from build123d import *

# Parameters (mm, degrees)
SKIZZE1_W                       = 1453
SKIZZE1_H                       = 700
SKIZZE1_W_2                     = 1333
SKIZZE1_H_2                     = 580
AUFSATZ_LINEAR_AUSTRAGEN1_DEPTH = 60
VERRUNDUNG1_R                   = 10
SKIZZE2_W                       = 300
SKIZZE2_H                       = 60
AUFSATZ_LINEAR_AUSTRAGEN2_DEPTH = 120
VERRUNDUNG3_R                   = 10
VERRUNDUNG4_R                   = 10
SKIZZE3_R                       = 8.75
SCHNITT_LINEAR_AUSTRAGEN1_DEPTH = 120
SKIZZE4_W                       = 80
SKIZZE4_H                       = 40
AUFSATZ_LINEAR_AUSTRAGEN3_DEPTH = 25


with BuildPart() as part:
    # Skizze1 → Aufsatz-Linear austragen1 (new, symmetric)
    with BuildSketch(Plane(origin=(0, 0, 0), x_dir=(1, 0, 0), z_dir=(0, 1, 0))):
        Rectangle(SKIZZE1_W, SKIZZE1_H)
        Rectangle(SKIZZE1_W_2, SKIZZE1_H_2, mode=Mode.SUBTRACT)
    extrude(amount=AUFSATZ_LINEAR_AUSTRAGEN1_DEPTH, both=True)

    # Verrundung1
    verrundung1_edges = [part.edges().sort_by_distance(p)[0] for p in [
        (726.5, 60, 0),
        (0, 60, -350),
        (-666.5, -60, 0),
        (0, -60, 290),
        (666.5, -60, 0),
        (0, -60, -290),
        (-666.5, 60, 0),
        (0, 60, 290),
        (666.5, 60, 0),
        (0, 60, -290),
        (-726.5, 60, 0),
        (0, -60, -350),
        (726.5, -60, 0),
        (0, -60, 350),
        (-726.5, -60, 0),
        (0, 60, 350),
    ]]
    fillet(verrundung1_edges, radius=VERRUNDUNG1_R)

    # Skizze2 → Aufsatz-Linear austragen2 (add)
    with BuildSketch(Plane.XZ.offset(60)):
        with Locations((-576.5, 320)):
            Rectangle(SKIZZE2_W, SKIZZE2_H)
        with Locations((576.5, 320)):
            Rectangle(SKIZZE2_W, SKIZZE2_H)
        with Locations((576.5, -320)):
            Rectangle(SKIZZE2_W, SKIZZE2_H)
        with Locations((-576.5, -320)):
            Rectangle(SKIZZE2_W, SKIZZE2_H)
    extrude(amount=AUFSATZ_LINEAR_AUSTRAGEN2_DEPTH)

    # Verrundung3
    verrundung3_edges = [part.edges().sort_by_distance(p)[0] for p in [
        (576.5, -180, 290),
        (576.5, -180, -290),
        (576.5, -180, -350),
        (-576.5, -180, -350),
        (-576.5, -180, -290),
        (-576.5, -180, 290),
        (-576.5, -180, 350),
        (576.5, -180, 350),
    ]]
    fillet(verrundung3_edges, radius=VERRUNDUNG3_R)

    # Verrundung4
    # the kernel refuses this fillet: 10 mm, written as the material it adds along each edge
    # the kernel refuses this fillet: 10 mm, written as the material it takes off along each edge
    with BuildSketch(Plane(origin=(691.5, -60, -290), x_dir=(0, 0, -1), z_dir=(1, 0, 0)), Plane(origin=(-691.5, -60, -290), x_dir=(0, -1, 0), z_dir=(-1, 0, 0))) as verrundung4_2_piece_1:
        with BuildLine():
            CenterArc((VERRUNDUNG4_R, -VERRUNDUNG4_R), VERRUNDUNG4_R, 90, 90)
            Line((0, -VERRUNDUNG4_R), (0, 0))
            Line((0, 0), (VERRUNDUNG4_R, 0))
        make_face()
    extrude(amount=60, mode=Mode.SUBTRACT)
    with BuildSketch(Plane(origin=(401.5, -60, -290), x_dir=(0, 0, -1), z_dir=(1, 0, 0)), Plane(origin=(-401.5, -60, -290), x_dir=(0, -1, 0), z_dir=(-1, 0, 0))) as verrundung4_2_piece_2:
        with BuildLine():
            CenterArc((VERRUNDUNG4_R, -VERRUNDUNG4_R), VERRUNDUNG4_R, 90, 90)
            Line((0, -VERRUNDUNG4_R), (0, 0))
            Line((0, 0), (VERRUNDUNG4_R, 0))
        make_face()
    extrude(amount=300, mode=Mode.SUBTRACT)
    with BuildSketch(Plane(origin=(751.5, -60, -350), x_dir=(0, 0, 1), z_dir=(-1, 0, 0)), Plane(origin=(-751.5, -60, 350), x_dir=(0, 0, -1), z_dir=(1, 0, 0))) as verrundung4_2_piece_3:
        with BuildLine():
            CenterArc((VERRUNDUNG4_R, -VERRUNDUNG4_R), VERRUNDUNG4_R, 90, 90)
            Line((0, -VERRUNDUNG4_R), (0, 0))
            Line((0, 0), (VERRUNDUNG4_R, 0))
        make_face()
    extrude(amount=350, mode=Mode.SUBTRACT)
    with BuildSketch(Plane(origin=(-751.5, -60, -350), x_dir=(0, 0, 1), z_dir=(1, 0, 0)), Plane(origin=(751.5, -60, 350), x_dir=(0, 0, -1), z_dir=(-1, 0, 0))) as verrundung4_2_piece_4:
        with BuildLine():
            CenterArc((VERRUNDUNG4_R, VERRUNDUNG4_R), VERRUNDUNG4_R, 180, 90)
            Line((0, VERRUNDUNG4_R), (0, 0))
            Line((0, 0), (VERRUNDUNG4_R, 0))
        make_face()
    extrude(amount=350, mode=Mode.SUBTRACT)
    with BuildSketch(Plane(origin=(-691.5, -60, 290), x_dir=(0, -1, 0), z_dir=(-1, 0, 0)), Plane(origin=(691.5, -60, 290), x_dir=(0, 0, 1), z_dir=(1, 0, 0))) as verrundung4_2_piece_5:
        with BuildLine():
            CenterArc((VERRUNDUNG4_R, VERRUNDUNG4_R), VERRUNDUNG4_R, 180, 90)
            Line((0, VERRUNDUNG4_R), (0, 0))
            Line((0, 0), (VERRUNDUNG4_R, 0))
        make_face()
    extrude(amount=60, mode=Mode.SUBTRACT)
    with BuildSketch(Plane(origin=(-401.5, -60, 290), x_dir=(0, -1, 0), z_dir=(-1, 0, 0)), Plane(origin=(401.5, -60, 290), x_dir=(0, 0, 1), z_dir=(1, 0, 0))) as verrundung4_2_piece_6:
        with BuildLine():
            CenterArc((VERRUNDUNG4_R, VERRUNDUNG4_R), VERRUNDUNG4_R, 180, 90)
            Line((0, VERRUNDUNG4_R), (0, 0))
            Line((0, 0), (VERRUNDUNG4_R, 0))
        make_face()
    extrude(amount=300, mode=Mode.SUBTRACT)

    # Skizze3 → Schnitt-Linear austragen1 (cut)
    with BuildSketch(Plane.XZ.offset(180)):
        with Locations(Location((-619.5, 320, 0), (0, 0, 270))):
            Circle(SKIZZE3_R)
        with Locations(Location((-619.5, -320, 0), (0, 0, 270))):
            Circle(SKIZZE3_R)
        with Locations(Location((619.5, 320, 0), (0, 0, 270))):
            Circle(SKIZZE3_R)
        with Locations(Location((619.5, -320, 0), (0, 0, 270))):
            Circle(SKIZZE3_R)
    extrude(amount=-SCHNITT_LINEAR_AUSTRAGEN1_DEPTH, mode=Mode.SUBTRACT)

    # Skizze4 → Aufsatz-Linear austragen3 (add)
    with BuildSketch(Plane.XZ.offset(180)):
        with Locations((-551.5, 320)):
            Rectangle(SKIZZE4_W, SKIZZE4_H)
        with Locations((551.5, 320)):
            Rectangle(SKIZZE4_W, SKIZZE4_H)
        with Locations((551.5, -320)):
            Rectangle(SKIZZE4_W, SKIZZE4_H)
        with Locations((-551.5, -320)):
            Rectangle(SKIZZE4_W, SKIZZE4_H)
    extrude(amount=AUFSATZ_LINEAR_AUSTRAGEN3_DEPTH)


solid = part.part
Verification items for the finished model (mm, model axes). A direction names the side the tool comes from. Coordinates: 2 decimals unless noted, no trailing zeros. Loops run counter-clockwise (first coordinate to the right, second up) from the corner with the lowest first, then second, coordinate; pieces in that order, holes last. Notation, with made-up numbers: (23, 7.25) -> (43, 7.25) arc R21 cw to (43, 13.25) -> close; hole circle Ø3 at (81, 36). An arc over 180 degrees is marked (long way). Answer as CSV lines item,"result".
1) Depth check by flat-ended pin: pin 1 (7.5 mm diameter, centred on y = -196, z = -321.5, fed in from -X); pin 2 (14 mm diameter, centred on x = -617.5, z = -317.5, fed in from -Y); pin 3 (20 mm diameter, centred on y = -194, z = 321, fed in from +X). Enter the tip coordinate at first touch or a pass-through.
Found:
pin 1,"stops at x = -591.5"
pin 2,"stops at y = -180"
pin 3,"stops at x = 591.5"
2) Cross-section at C-C, the plane z = -50.5. Record the cut outline in (x, y).
Found:
outline,"(-726.5, -50) arc R10 ccw to (-716.5, -60) -> (-676.5, -60) arc R10 ccw to (-666.5, -50) -> (-666.5, 50) arc R10 ccw to (-676.5, 60) -> (-716.5, 60) arc R10 ccw to (-726.5, 50) -> close; (666.5, -50) arc R10 ccw to (676.5, -60) -> (716.5, -60) arc R10 ccw to (726.5, -50) -> (726.5, 50) arc R10 ccw to (716.5, 60) -> (676.5, 60) arc R10 ccw to (666.5, 50) -> close"
3) Cross-section at A-A, the plane y = -151.5. Record the cut outline in (x, z), then the cut area to 3 significant figures.
Found:
outline,"(-726.5, -350) -> (-426.5, -350) -> (-426.5, -290) -> (-726.5, -290) -> close; (-726.5, 290) -> (-426.5, 290) -> (-426.5, 350) -> (-726.5, 350) -> close; (426.5, -350) -> (726.5, -350) -> (726.5, -290) -> (426.5, -290) -> close; (426.5, 290) -> (726.5, 290) -> (726.5, 350) -> (426.5, 350) -> close; hole circle Ø17.5 at (-619.5, -320); hole circle Ø17.5 at (-619.5, 320); hole circle Ø17.5 at (619.5, -320); hole circle Ø17.5 at (619.5, 320)"
area,"71,000 mm2"
4) Thickness scan on L1, parallel to X at y = -142, z = 320; L2, parallel to Z at x = -619, y = -96; L3, parallel to Z at x = 242, y = -6. Record the ranges inside material, lowest first. Write a range as from..to.
Found:
L1,"x = -726.5..-628.25, -610.75..-426.5, 426.5..610.75, 628.25..726.5"
L2,"z = -350..-328.74, -311.26..-290, 290..311.26, 328.74..350"
L3,"z = -350..-290, 290..350"
5) Tool access check on faces 5 (the flat face through (591.5, -192, -320)), 6 (the flat face through (-660, -180, 320)), 7 (the flat face through (574, -119, -290)), 8 (the flat face through (551, -192, 340)), 9 (the flat face through (-552, -192, -340)). Record the directions out of +Z, -Z, +X, -X, +Y, -Y that give a thin tool (end or side, any length) a straight path to the whole face; none if there is none.
Found:
face 5,"+Z, -Z, +X, -Y"
face 6,"+Z, -Z, -X, -Y"
face 7,"+X, -X, -Y"
face 8,"+Z, +X, -X, -Y"
face 9,"-Z, +X, -X, -Y"
6) Release check for a two-part mould opening along X. For faces 1 (the flat face through (-426.5, -119, -320)), 2 (the flat face through (-726.5, -119, -320)), 3 (the flat face through (-6, -60, -320)), 4 (the flat face through (-696, -60, 4)) record: +X half, -X half, draft (parallel to the pull), parting line (faces both ways), or undercut.
Found:
face 1,"undercut"
face 2,"-X half"
face 3,"undercut"
face 4,"draft"
7) Cross-section at D-D, the plane y = 14. Record the cut outline in (x, z), then the cut area to 3 significant figures.
Found:
outline,"(-726.5, -350) -> (726.5, -350) -> (726.5, 350) -> (-726.5, 350) -> close; hole (-666.5, -290) -> (666.5, -290) -> (666.5, 290) -> (-666.5, 290) -> close"
area,"244,000 mm2"
8) Cross-section at B-B, the plane x = -323. Record the cut outline in (y, z).
Found:
outline,"(-60, -340) arc R10 ccw to (-50, -350) -> (50, -350) arc R10 ccw to (60, -340) -> (60, -300) arc R10 ccw to (50, -290) -> (-50, -290) arc R10 ccw to (-60, -300) -> close; (-60, 300) arc R10 ccw to (-50, 290) -> (50, 290) arc R10 ccw to (60, 300) -> (60, 340) arc R10 ccw to (50, 350) -> (-50, 350) arc R10 ccw to (-60, 340) -> close"
